Verification items for the finished model (mm, model axes). A direction names the side the tool comes from. Coordinates: 2 decimals unless noted, no trailing zeros. Write each loop counter-clockwise with the first axis right and the second up, starting at its lowest first coordinate (ties: lowest second). Pieces come first, ordered by that corner, then holes. Notation, with made-up numbers: M -13,-25.75 L 8,-25.75 A17 ccw 8,-6.75 Z; hole C -1,72 d5. An arc over 180 degrees is marked long. Answer in a Markdown table with one row per item.
from build123d import *

# Parameters (mm, degrees)
SKETCH_1_R      = 1.45
EXTRUDE_1_DEPTH = 2
FILLET_2_R      = 3


with BuildPart() as part:
    # 草图1 → 凸台-拉伸1 (new body)
    with BuildSketch(Plane(origin=(0, 0, 0), x_dir=(1, 0, 0), z_dir=(0, 1, 0))):
        Polygon((15, 28), (43, 0), (43, -15), (0, -15), (0, 0), (0, 28), align=None)
        with Locations(Location((24.5, -7.5, 0), (0, 0, 270))):
            Circle(SKETCH_1_R, mode=Mode.SUBTRACT)
        with Locations(Location((7.5, 9.5, 0), (0, 0, 270))):
            Circle(SKETCH_1_R, mode=Mode.SUBTRACT)
        with Locations(Location((38, -7.5, 0), (0, 0, 270))):
            Circle(SKETCH_1_R, mode=Mode.SUBTRACT)
        with Locations(Location((7.5, 23, 0), (0, 0, 270))):
            Circle(SKETCH_1_R, mode=Mode.SUBTRACT)
        Polygon((15, 20.928932188), (35.928932188, 0), (15, 0), align=None, mode=Mode.SUBTRACT)
    extrude(amount=EXTRUDE_1_DEPTH)

    # 圆角2
    fillet_2_edges = [part.edges().sort_by_distance(p)[0] for p in [
        (0, 1, -28),
        (15, 1, -28),
        (43, 1, 0),
        (43, 1, 15),
        (0, 1, 15),
        (15, 1, -20.928932188),
        (15, 1, 0),
        (35.928932188, 1, 0),
    ]]
    fillet(fillet_2_edges, radius=FILLET_2_R)


solid = part.part
1) Thickness scan on L1, parallel to X at y = 0.9, z = 7.5; L2, parallel to X at y = 1.6, z = -15; L3, parallel to Z at x = 25.5, y = 0.7. Record the ranges inside material, lowest first. Write a range as [from, to].
Response values:
| item | result |
|---|---|
| L1 | x = [0, 23.05], [25.95, 36.55], [39.45, 43] |
| L2 | x = [0, 15.3], [20.93, 28] |
| L3 | z = [-17.5, -10.43], [0, 6.45], [8.55, 15] |
2) Release check for a two-part mould opening along X. For faces 3 (the face through (43, 1, 7)), 4 (the face through (6.62, 0.99, -10.65)), 5 (the face through (0.9, 1.01, -27.14)) record: +X half, -X half, draft (parallel to the pull), parting line (faces both ways), or undercut.
Response values:
| item | result |
|---|---|
| face 3 | +X half |
| face 4 | undercut |
| face 5 | -X half |
3) Depth check by flat-ended pin: pin 1 (4.5 mm diameter, centred on x = 7.5, z = -9.5, fed in from -Y). Enter the tip coordinate at first touch or a pass-through.
Response values:
| item | result |
|---|---|
| pin 1 | stops at y = 0 |
4) Sectioned sample at D-D (x = 38). Record the cut outline in (y, z).
Response values:
| item | result |
|---|---|
| outline | M 0,-5 L 2,-5 L 2,6.05 L 0,6.05 Z; M 0,8.95 L 2,8.95 L 2,15 L 0,15 Z |
5) Sectioned sample at A-A (z = -23). Record the cut outline in (x, y), then the cut area to 3 significant figures.
Response values:
| item | result |
|---|---|
| outline | M 0,0 L 6.05,0 L 6.05,2 L 0,2 Z; M 8.95,0 L 20,0 L 20,2 L 8.95,2 Z |
| area | 34.2 mm² |
6) Tool access check on faces 1 (the face through (15, 1, -8)), 2 (the face through (0.86, 1.01, 14.1)). Record the directions out of +Z, -Z, +X, -X, +Y, -Y that give a thin tool (end or side, any length) a straight path to the whole face; none if there is none.
Response values:
| item | result |
|---|---|
| face 1 | +Y, -Y |
| face 2 | +Z, -X, +Y, -Y |
7) Sectioned sample at B-B (x = 7.5). Record the cut outline in (y, z), then the cut area to 3 significant figures.
Response values:
| item | result |
|---|---|
| outline | M 0,-28 L 2,-28 L 2,-24.45 L 0,-24.45 Z; M 0,-21.55 L 2,-21.55 L 2,-10.95 L 0,-10.95 Z; M 0,-8.05 L 2,-8.05 L 2,15 L 0,15 Z |
| area | 74.4 mm² |
8) Sectioned sample at C-C (z = 7.5). Record the cut outline in (x, y).
Response values:
| item | result |
|---|---|
| outline | M 0,0 L 23.05,0 L 23.05,2 L 0,2 Z; M 25.95,0 L 36.55,0 L 36.55,2 L 25.95,2 Z; M 39.45,0 L 43,0 L 43,2 L 39.45,2 Z |
